The model under review builds one solid part; all positions refer to its coordinate system, in mm. A direction names the side the tool comes from. Round coordinates to 2 decimals unless told otherwise and drop trailing zeros. Write each loop counter-clockwise with the first axis right and the second up, starting at its lowest first coordinate (ties: lowest second). Pieces come first, ordered by that corner, then holes. Notation, with made-up numbers: M 14.5,87 L 56.5,87 A12 ccw 56.5,106 Z; hole C 88,15 d1. An arc over 180 degrees is marked long. Write item = value, one per line. Start each with the question number.
Item 1: Take a section at A-A, the plane y = 0. Give the boundary of the cut face in (x, z), plus the area to 3 significant figures.
Item 2: Take a section at B-B, the plane z = 0. Give the boundary of the cut face in (x, y), plus the area to 3 significant figures.
Item 3: Tool access review of faces 1 (the flat face through (0, 3.4, 1.9)), 2 (the flat face through (8.738, -2, 0)), 3 (the flat face through (-2.388, -5, -3)): name each direction out of +Z, -Z, +X, -X, +Y, -Y from which nothing blocks a thin tool from reaching the whole face with its end or side.
Item 4: The part is to be moulded in two halves that separate along Z. For faces 4 (the cylindrical face through (0.122, 0.966, -1.26)), 5 (the flat face through (-8.738, -1.3, 1.2)), 6 (the cylindrical face through (-5.607, -1.671, 5.306)), say which applies: +Z half, -Z half, draft (parallel to the pull), parting line (faces both ways), or undercut.
Item 5: To check wall thickness, follow line 1 along Y through (x, z) = (-3.5, 0); line 2 along X through (y, z) = (-2.5, 4.25); line 3 along Y through (x, z) = (3.25, 0). State the ranges of each line that lie inside material, in increasing order.
Item 6: Take a section at C-C, the plane x = -3. Give the boundary of the cut face in (y, z) (1 decimal), plus the area to 3 significant figures.
Item 7: For pin 1 Ø8 at (x, z) = (-3.5, -4) entering from -Y; pin 2 Ø5 at (x, z) = (-6.5, -2) entering from +Y; pin 3 Ø1 at (x, z) = (-6, -3.5) entering from +Y, all flat-tipped, find the tip position at first contact; note any pin that passes through.
from build123d import *

# Parameters (mm, degrees)
SKETCH4_R          = 4.5339
SKETCH4_R_2        = 4.37515
CUT_EXTRUDE2_DEPTH = 6.35
CUT_EXTRUDE1_DEPTH = 6.35
CIRPATTERN1_COUNT  = 14


with BuildPart() as part:
    # Sketch1 → Revolve1 (revolve)
    with BuildSketch(Plane.XY, mode=Mode.PRIVATE) as revolve1_sk:
        with BuildLine():
            Line((-8.7376, 1.5875), (8.7376, 1.5875))
            Line((8.7376, 1.5875), (8.7376, 6.731))
            Line((8.7376, 6.731), (7.5438, 6.731))
            ThreePointArc((7.5438, 6.731), (6.680508602, 6.113831183), (6.35, 5.1054))
            Line((6.35, 5.1054), (6.35, 4.5339))
            Line((6.35, 4.5339), (0, 4.5339))
            Line((0, 4.5339), (0, 5.1054))
            ThreePointArc((0, 5.1054), (-0.330508602, 6.113831183), (-1.1938, 6.731))
            Line((-1.1938, 6.731), (-2.3876, 6.731))
            Line((-2.3876, 6.731), (-2.3876, 5.5626))
            Line((-2.3876, 5.5626), (-8.7376, 5.5626))
            Line((-8.7376, 5.5626), (-8.7376, 1.5875))
        make_face()
    revolve(revolve1_sk.sketch.rotate(Axis((-8.7376, 0, 0), (1, 0, 0)), 90), axis=Axis((-8.7376, 0, 0), (1, 0, 0)))

    # Sketch4 → Cut-Extrude2 (cut)
    with BuildSketch(Plane(origin=(0, 0, 0), x_dir=(0, 0, -1), z_dir=(1, 0, 0))):
        Circle(SKETCH4_R)
        Circle(SKETCH4_R_2, mode=Mode.SUBTRACT)
    extrude(amount=CUT_EXTRUDE2_DEPTH, mode=Mode.SUBTRACT)

    # Sketch3 → Cut-Extrude1 (cut)
    with BuildSketch(Plane(origin=(0, 0, 0), x_dir=(0, 0, -1), z_dir=(1, 0, 0))):
        with BuildLine():
            Line((-0.641613493, 4.327848154), (-0.345249615, 3.692293767))
            Line((-0.345249615, 3.692293767), (0.345249615, 3.692293767))
            Line((0.345249615, 3.692293767), (0.641613493, 4.327848154))
            ThreePointArc((0.641613493, 4.327848154), (0, 4.37515), (-0.641613493, 4.327848154))
        make_face()
    cut_extrude1 = extrude(amount=CUT_EXTRUDE1_DEPTH, mode=Mode.SUBTRACT)

    # CirPattern1: Cut-Extrude1 ×14 about axis
    cirpattern1_axis = Axis((0, 0, 0), (1, 0, 0))
    for i in range(1, CIRPATTERN1_COUNT):
        add(cut_extrude1.rotate(cirpattern1_axis, i * 360 / CIRPATTERN1_COUNT), mode=Mode.SUBTRACT)


solid = part.part
Response values:
q1.outline = M -8.74,-5.56 L -2.39,-5.56 L -2.39,-6.73 L -1.19,-6.73 A1.7 ccw 0,-5.11 L 0,-4.38 L 6.35,-4.38 L 6.35,-5.11 A1.7 ccw 7.54,-6.73 L 8.74,-6.73 L 8.74,-1.59 L -8.74,-1.59 Z; M -8.74,1.59 L 8.74,1.59 L 8.74,6.73 L 7.54,6.73 A1.7 ccw 6.35,5.11 L 6.35,4.38 L 0,4.38 L 0,5.11 A1.7 ccw -1.19,6.73 L -2.39,6.73 L -2.39,5.56 L -8.74,5.56 Z
q1.area = 133 mm2
q2.outline = M -8.74,-5.56 L -2.39,-5.56 L -2.39,-6.73 L -1.19,-6.73 A1.7 ccw 0,-5.11 L 0,-3.69 L 6.35,-3.69 L 6.35,-5.11 A1.7 ccw 7.54,-6.73 L 8.74,-6.73 L 8.74,-1.59 L -8.74,-1.59 Z; M -8.74,1.59 L 8.74,1.59 L 8.74,6.73 L 7.54,6.73 A1.7 ccw 6.35,5.11 L 6.35,3.69 L 0,3.69 L 0,5.11 A1.7 ccw -1.19,6.73 L -2.39,6.73 L -2.39,5.56 L -8.74,5.56 Z
q2.area = 124 mm2
q3.face_1 = none
q3.face_2 = +Z, -Z, +X, +Y, -Y
q3.face_3 = -X
q4.face_4 = undercut
q4.face_5 = draft
q4.face_6 = parting line
q5.line_1 = -5.56 to -1.59, 1.59 to 5.56
q5.line_2 = -8.74 to 0, 6.35 to 8.74
q5.line_3 = -3.69 to -1.59, 1.59 to 3.69
q6.outline = C 0,0 d11.1; hole C 0,0 d3.2
q6.area = 89.3 mm2
q7.pin_1 = -6.73
q7.pin_2 = 5.56
q7.pin_3 = 4.68
